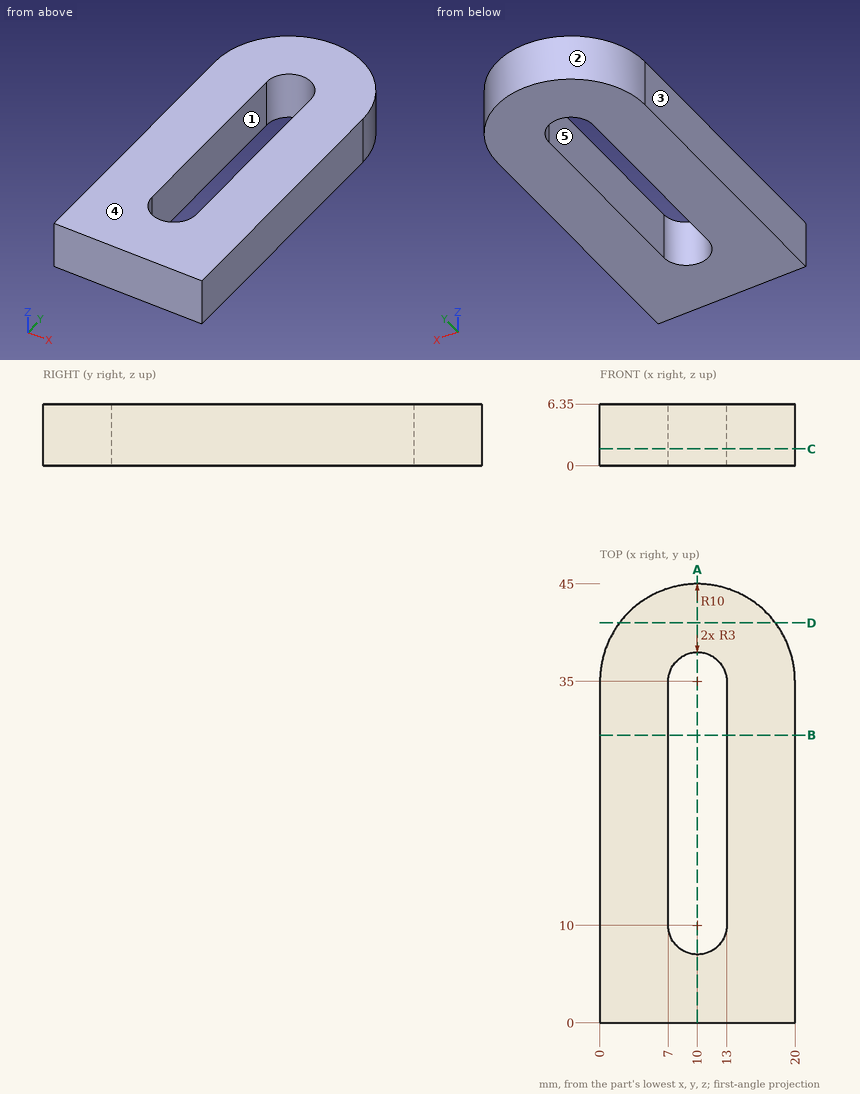
Design review of the part shown in the three views and the two pictorial views. Dimensions are in mm from the part's minimum x, y and z. A direction names the side the tool comes from. Coordinates: 2 decimals unless noted, no trailing zeros. Order: outer loops, then holes, each group sorted by start corner. A loop starts at its lowest first (then second) coordinate and runs counter-clockwise, first axis right, second up.
1) Take a section at A-A, the plane x = 10. Give the boundary of the cut face in (y, z), and give its area (3 significant figures).
2) Clearance check with a flat-ended pin moving along its axis: pin 1 (1.5 mm diameter, centred on y = 16.5, z = 2, fed in from -X). State where the tip first meets the part, or that it passes through.
3) For the marked faces 4 and 5, list the 3-axis set-ups (+Z, -Z, +X, -X, +Y, -Y) from which the entire face can be reached by the end or side of a thin tool; tool diameter is ignored.
4) Wall thickness on line 1 along X through (y, z) = (21.5, 4.5); line 2 along Y through (x, z) = (10, 6.25); line 3 along Y through (x, z) = (8.5, 0.5): over which ranges is each line inside the solid? List them lowest first.
5) Take a section at D-D, the plane y = 41. Give the boundary of the cut face in (x, z), and give its area (3 significant figures).
6) Take a section at B-B, the plane y = 29.5. Give the boundary of the cut face in (x, z), and give its area (3 significant figures).
7) Take a section at C-C, the plane z = 1.75. Give the boundary of the cut face in (x, y), and give its area (3 significant figures).
8) Mouldability with a two-part tool opening along X and no side actions: class the marked faces 1, 2 and 3 as +X half, -X half, draft (parallel to the pull), parting line (faces both ways), or undercut.
Returned:
1. outline: (0, 0) - (7, 0) - (7, 6.35) - (0, 6.35) - close; (38, 0) - (45, 0) - (45, 6.35) - (38, 6.35) - close
1. area: 88.9 mm2
2. pin 1: stops at x = 0
3. face 4: +Z, +X, -X, +Y, -Y
3. face 5: +Z, -Z
4. line 1: x = 0 to 7, 13 to 20
4. line 2: y = 0 to 7, 38 to 45
4. line 3: y = 0 to 7.4, 37.6 to 44.89
5. outline: (2, 0) - (18, 0) - (18, 6.35) - (2, 6.35) - close
5. area: 102 mm2
6. outline: (0, 0) - (7, 0) - (7, 6.35) - (0, 6.35) - close; (13, 0) - (20, 0) - (20, 6.35) - (13, 6.35) - close
6. area: 88.9 mm2
7. outline: (0, 0) - (20, 0) - (20, 35) arc R10 ccw to (0, 35) - close; hole (7, 10) arc R3 ccw to (13, 10) - (13, 35) arc R3 ccw to (7, 35) - close
7. area: 679 mm2
8. face 1: undercut
8. face 2: parting line
8. face 3: -X half
